from build123d import *

# Parameters (mm, degrees)
F0_W     = 36.2096428871
F0_H     = 33.7809510529
F1_DEPTH = 50
F2_W     = 32.2096428871
F2_H     = 46
F3_DEPTH = 32
F4_SIZE  = 2


with BuildPart() as f1:
    # F0 (on Front) → F1 (new body)
    with BuildSketch(Plane.XZ):
        with Locations((18.1048214436, 16.8904755265)):
            Rectangle(F0_W, F0_H)
    extrude(amount=F1_DEPTH)

    # F2 (on face) → F3 (cut)
    with BuildSketch(Plane.XY.offset(33.7809510529)):
        with Locations((18.1048214436, -25)):
            Rectangle(F2_W, F2_H)
    extrude(amount=-F3_DEPTH, mode=Mode.SUBTRACT)

    # F4
    f4_edges = [f1.edges().sort_by_distance(p)[0] for p in [
        (18.104821, 0, 0),
        (0, -25, 0),
        (36.209643, -25, 0),
        (18.104821, -50, 0),
    ]]
    chamfer(f4_edges, length=F4_SIZE)


solid = f1.part
Check sheet for the modelled part. Datum: model origin and axes. Units: mm. A direction names the side the tool comes from. Give positions to 0.01 mm unless a question says otherwise; leave off trailing zeros. Loops run counter-clockwise (first coordinate to the right, second up) from the corner with the lowest first, then second, coordinate; pieces in that order, holes last. Notation, with made-up numbers: M -15,31.5 L 29,31.5 A23 cw 29,52.5 Z; hole C -38.5,4.5 d7. An arc over 180 degrees is marked long. Answer as a JSON object with one key per item and string values. Group by question number.
Q1. Go/stop test with flat-tipped pins: P1, Ø1, axis at x = 17, y = -29, coming from the +Z side; P2, Ø10, axis at x = 6.5, y = -22.5, coming from the +Z side. Record where each tip stops, or that it passes through.
Q2. Material ranges on line 1 along X through (y, z) = (-11, 31.5); line 2 along Y through (x, z) = (24.5, 16); line 3 along Z through (x, y) = (20, -35), recorded low to high. Write a range as [from, to].
Q3. Access from +Z, -Z, +X, -X, +Y, -Y to the whole of each face (thin tool, end or side, straight path). Record for faces 4 (the flat face through (34.21, -25, 18)), 5 (the flat face through (0, -25, 18)).
Q4. Cross-section at A-A on z = 17.5. Record the cut outline in (x, y), then the cut area to 3 significant figures.
Q5. Release check for a two-part mould opening along Y. For faces 1 (the flat face through (18, -50, 18)), 2 (the flat face through (18, -2, 18)), 3 (the flat face through (1, -27, 33.781)) record: released by +Y, released by -Y, zero draft, split by the parting line, or undercut.
Q6. Cross-section at C-C on y = -34. Record the cut outline in (x, z), then the cut area to 3 significant figures.
Q7. Cross-section at B-B on x = 21.5. Record the cut outline in (y, z).
Evaluation:
{
 "1": {"P1": "stops at z = 1.78", "P2": "stops at z = 33.78"},
 "2": {"line 1": "x = [0, 2], [34.21, 36.21]", "line 2": "y = [-50, -48], [-2, 0]", "line 3": "z = [0, 1.78]"},
 "3": {"face 4": "+Z", "face 5": "+Z, -Z, -X, +Y, -Y"},
 "4": {"outline": "M 0,-50 L 36.21,-50 L 36.21,0 L 0,0 Z; hole M 2,-48 L 34.21,-48 L 34.21,-2 L 2,-2 Z", "area": "329 mm2"},
 "5": {"face 1": "released by -Y", "face 2": "undercut", "face 3": "zero draft"},
 "6": {"outline": "M 0,2 L 2,0 L 34.21,0 L 36.21,2 L 36.21,33.78 L 34.21,33.78 L 34.21,1.78 L 2,1.78 L 2,33.78 L 0,33.78 Z", "area": "188 mm2"},
 "7": {"outline": "M -50,2 L -48,0 L -2,0 L 0,2 L 0,33.78 L -2,33.78 L -2,1.78 L -48,1.78 L -48,33.78 L -50,33.78 Z"}
}
